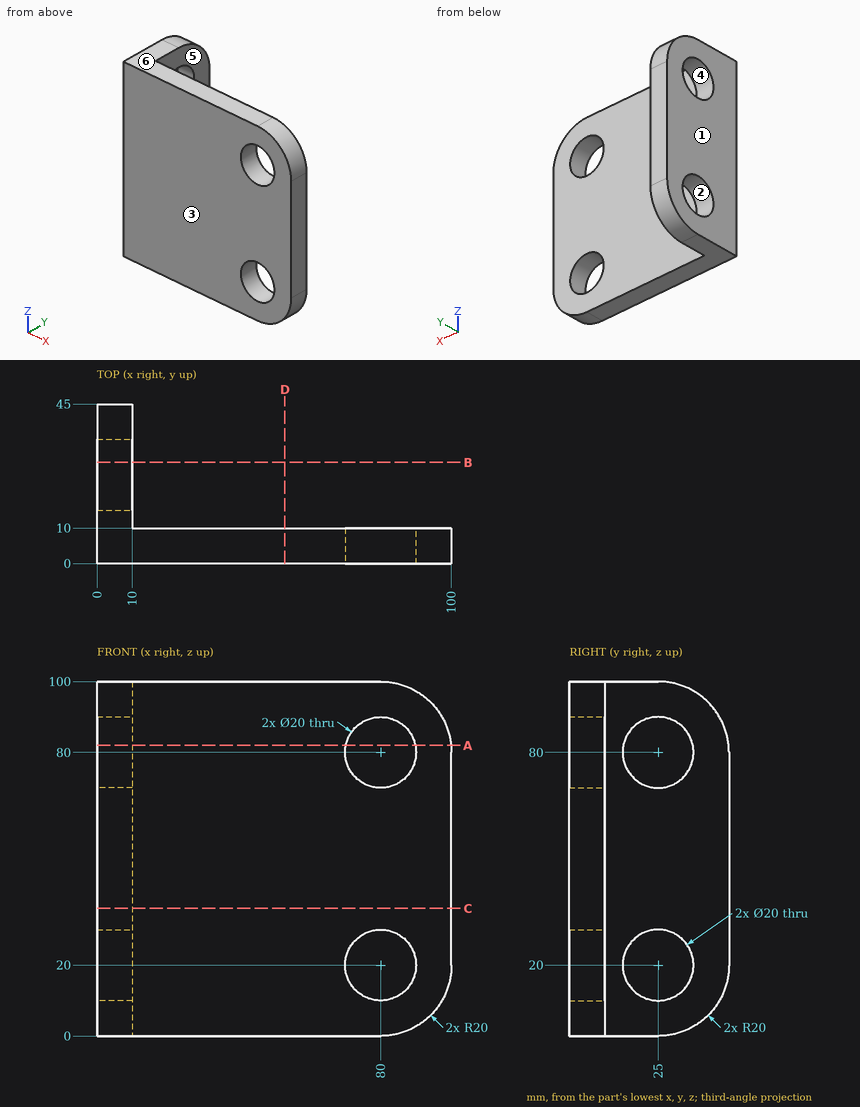
Input: dimensioned drawing with shaded views. Units: mm. Origin: part minimum x, y, z. A direction names the side the tool comes from. Coordinates: 2 decimals unless noted, no trailing zeros. Write each loop counter-clockwise with the first axis right and the second up, starting at its lowest first coordinate (ties: lowest second). Pieces come first, ordered by that corner, then holes. Notation, with made-up numbers: M -32,39.5 L -19,39.5 A27 cw -19,58.5 Z; hole C 42.5,42.25 d5. An arc over 180 degrees is marked long. Answer as a JSON object with one key per item and string values. Group by question number.
(1) Section D-D on x = 53. Output: boundary loops of the cut face in (y, z), plus the area to 3 significant figures.
(2) Ray query, line 1 along Z through (x, y) = (80, 5); line 2 along X through (y, z) = (36, 46). Return the intervals inside material, ascending. Write a range as [from, to].
(3) Mould query, pull axis Y, two halves, no side actions, for the marked faces 1, 2, 3 and 4. Classes: pulls with the +Y half, pulls with the -Y half, needs draft (parallel to the pull), parting line crosses it, or undercut.
(4) Section C-C on z = 36. Output: boundary loops of the cut face in (x, y), plus the area to 3 significant figures.
(5) Set-up query: the marked faces 5 and 6. Return all of +Z, -Z, +X, -X, +Y, -Y with unobstructed straight access to the full face (end or side cutting, diameter ignored); none if empty.
(6) Section B-B on y = 28.5. Output: boundary loops of the cut face in (x, z), plus the area to 3 significant figures.
(7) Contact query for flat-ended pins moving along their axis: P1, Ø3, axis at x = 34.5, z = 38.5, coming from the +Y side; P2, Ø5, axis at y = 5, z = 27, coming from the -X side; P3, Ø1.5, axis at x = 61.5, y = 12, coming from the -Z side; P4, Ø17.5, axis at y = 21, z = 28.5, coming from the +X side. Output: stop coordinate, or through.
(8) Section A-A on z = 82. Output: boundary loops of the cut face in (x, y), plus the area to 3 significant figures.
Result set:
{
 "1": {"outline": "M 0,0 L 10,0 L 10,100 L 0,100 Z", "area": "1,000 mm2"},
 "2": {"line 1": "z = [0, 10], [30, 70], [90, 100]", "line 2": "x = [0, 10]"},
 "3": {"face 1": "needs draft", "face 2": "undercut", "face 3": "pulls with the -Y half", "face 4": "undercut"},
 "4": {"outline": "M 0,0 L 100,0 L 100,10 L 10,10 L 10,45 L 0,45 Z", "area": "1,350 mm2"},
 "5": {"face 5": "+Z, -Z, +X, +Y", "face 6": "+Z, +X, -X, +Y, -Y"},
 "6": {"outline": "M 0,0.31 L 10,0.31 L 10,10.63 L 0,10.63 Z; M 0,29.37 L 10,29.37 L 10,70.63 L 0,70.63 Z; M 0,89.37 L 10,89.37 L 10,99.69 L 0,99.69 Z", "area": "619 mm2"},
 "7": {"P1": "stops at y = 10", "P2": "stops at x = 0", "P3": "passes through", "P4": "stops at x = 10"},
 "8": {"outline": "M 0,0 L 70.2,0 L 70.2,10 L 10,10 L 10,15.2 L 0,15.2 Z; M 0,34.8 L 10,34.8 L 10,44.9 L 0,44.9 Z; M 89.8,0 L 99.9,0 L 99.9,10 L 89.8,10 Z", "area": "956 mm2"}
}
